Geometry: see drawing. Coordinates: mm, zero at the bounding-box minimum. A direction names the side the tool comes from. Coordinates: 2 decimals unless noted, no trailing zeros. Write each loop counter-clockwise with the first axis right and the second up, starting at its lowest first coordinate (ties: lowest second). Pieces come first, ordered by that corner, then holes.
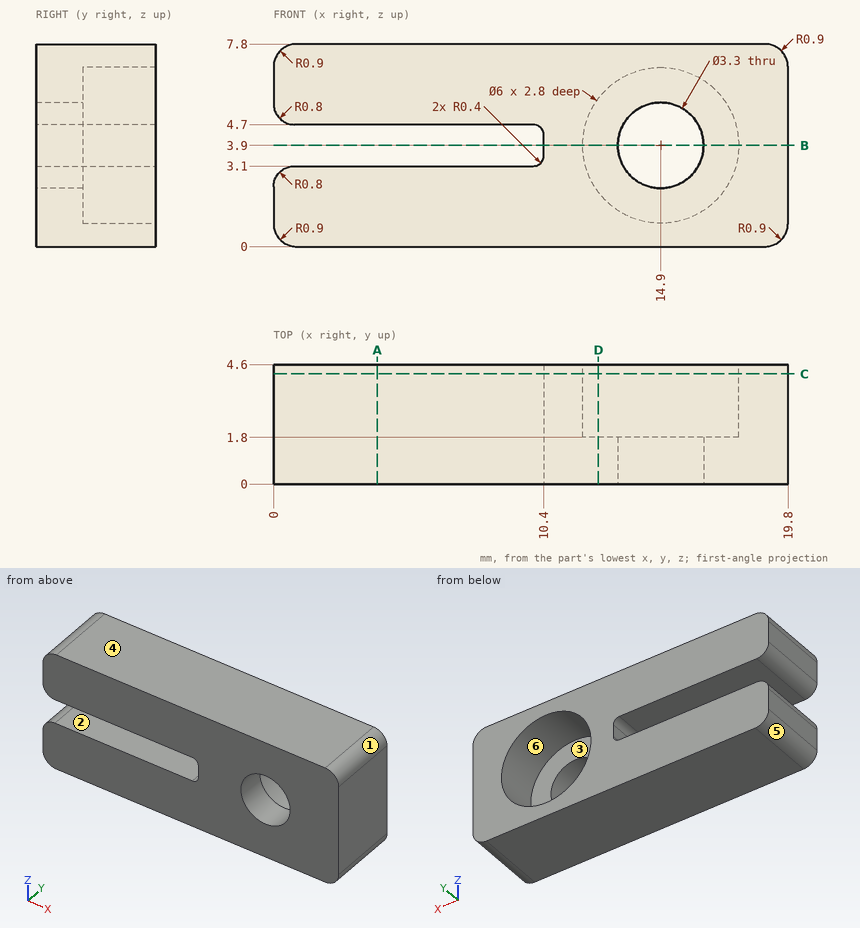
Item 1: Section D-D, the plane x = 12.5. Output: boundary loops of the cut face in (y, z).
Derived:
outline: (0, 0) - (4.6, 0) - (4.6, 2.1) - (1.8, 2.1) - (1.8, 5.7) - (4.6, 5.7) - (4.6, 7.8) - (0, 7.8) - close
Item 2: Pin query (flat end, axial travel): pin 1 (1.5 mm diameter, centred on x = 5, z = 4.5, fed in from -Y); pin 2 (2 mm diameter, centred on x = 14.9, z = 3.9, fed in from -Y). Return the tip coordinate at first contact, or that it passes through.
Derived:
pin 1: stops at y = 0
pin 2: passes through
Item 3: Section C-C, the plane y = 4.25. Output: boundary loops of the cut face in (x, z), plus the area to 3 significant figures.
Derived:
outline: (0, 0.9) arc R0.9 ccw to (0.9, 0) - (18.9, 0) arc R0.9 ccw to (19.8, 0.9) - (19.8, 6.9) arc R0.9 ccw to (18.9, 7.8) - (0.9, 7.8) arc R0.9 ccw to (0, 6.9) - (0, 5.5) arc R0.8 ccw to (0.8, 4.7) - (10, 4.7) arc R0.4 cw to (10.4, 4.3) - (10.4, 3.5) arc R0.4 cw to (10, 3.1) - (0.8, 3.1) arc R0.8 ccw to (0, 2.3) - close; hole circle Ø6 at (14.9, 3.9)
area: 109 mm2
Item 4: Material intervals for probe 1 along X at (y, z) = (3.9, 3.75); probe 2 along Z at (x, y) = (4, 2.4); probe 3 along X at (y, z) = (1, 3.9), sorted ascending.
Derived:
probe 1: x = 10.4 to 11.9, 17.9 to 19.8
probe 2: z = 0 to 3.1, 4.7 to 7.8
probe 3: x = 10.4 to 13.25, 16.55 to 19.8
Item 5: Section B-B, the plane z = 3.9. Output: boundary loops of the cut face in (x, y), plus the area to 3 significant figures.
Derived:
outline: (10.4, 0) - (13.25, 0) - (13.25, 1.8) - (11.9, 1.8) - (11.9, 4.6) - (10.4, 4.6) - close; (16.55, 0) - (19.8, 0) - (19.8, 4.6) - (17.9, 4.6) - (17.9, 1.8) - (16.55, 1.8) - close
area: 20.5 mm2
Item 6: Section A-A, the plane x = 4. Output: boundary loops of the cut face in (y, z).
Derived:
outline: (0, 0) - (4.6, 0) - (4.6, 3.1) - (0, 3.1) - close; (0, 4.7) - (4.6, 4.7) - (4.6, 7.8) - (0, 7.8) - close
Item 7: Set-up query: the marked faces 1, 2 and 3. Return all of +Z, -Z, +X, -X, +Y, -Y with unobstructed straight access to the full face (end or side cutting, diameter ignored); none if empty.
Derived:
face 1: +Z, +X, +Y, -Y
face 2: -X, +Y, -Y
face 3: +Y
Item 8: Pull-direction query (Z, two-part tool) for the marked faces 4, 5 and 6; classes: released by +Z, released by -Z, zero draft, split by the parting line, or undercut.
Derived:
face 4: released by +Z
face 5: released by -Z
face 6: undercut
